```python
from build123d import *
from build123d.topology import SkipClean

# Parameters (mm, degrees)
ESQUISSE2_R             = 11
BOSS_EXTRU_1_DEPTH      = 20
ENL_V_START             = -10
ESQUISSE3_R             = 12
ESQUISSE3_R_2           = 11
ENL_V_MAT_EXTRU_1_DEPTH = 10
ESQUISSE4_W             = 3
ESQUISSE4_H             = 10
BOSS_EXTRU_2_DEPTH      = 4
ESQUISSE5_R             = 1.1
BOSS_EXTRU_3_DEPTH      = 1
ESQUISSE9_R             = 1.1
BOSS_EXTRU_5_DEPTH      = 2
BOSS_EXTRU_6_START      = -6
BOSS_EXTRU_6_DEPTH      = 8
CONG_1_R                = 1
CONG_2_R                = 1
BOSS_EXTRU_7_DEPTH      = 10
BOSS_EXTRU_8_DEPTH      = 10
BOSS_EXTRU_8_DEPTH_BACK = 5
CONG_3_R                = 10
CONG_4_R                = 3
ENL_V_MAT_EXTRU_2_REACH = 52.872
ESQUISSE11_R            = 3


with BuildPart() as part:
    # Esquisse2 → Boss.-Extru.1 (new body)
    with BuildSketch(Plane.XY):
        with BuildLine():
            Line((5.727272727, 12.774910845), (24.045454545, 4.562468159))
            ThreePointArc((24.045454545, 4.562468159), (27, 0), (24.045454545, -4.562468159))
            Line((24.045454545, -4.562468159), (5.727272727, -12.774910845))
            ThreePointArc((5.727272727, -12.774910845), (-14, 0), (5.727272727, 12.774910845))
        make_face()
        Circle(ESQUISSE2_R, mode=Mode.SUBTRACT)
    extrude(amount=BOSS_EXTRU_1_DEPTH)

    # Esquisse3 → Enlèv. mat.-Extru.1 (cut)
    with BuildSketch(Plane.XY.offset(20).offset(ENL_V_START)):
        Circle(ESQUISSE3_R)
        Circle(ESQUISSE3_R_2, mode=Mode.SUBTRACT)
    extrude(amount=ENL_V_MAT_EXTRU_1_DEPTH, mode=Mode.SUBTRACT)

    # Esquisse4 → Boss.-Extru.2 (add)
    with BuildSketch(Plane(origin=(5.727272727, -12.774910845, 0), x_dir=(0.9124936318129423, 0.4090909090909094, 0), z_dir=(0.40909090909090934, -0.9124936318129422, 0))):
        with Locations((17.5748599, 10)):
            Rectangle(ESQUISSE4_W, ESQUISSE4_H)
    extrude(amount=BOSS_EXTRU_2_DEPTH)

    # Esquisse5 → Boss.-Extru.3 (add)
    with BuildSketch(Plane.XY.offset(15)):
        with Locations(Location((22.582402284, -7.410182695, 0), (0, 0, 180))):
            Circle(ESQUISSE5_R)
    boss_extru_3 = extrude(amount=BOSS_EXTRU_3_DEPTH)

    # Symétrie1: Boss.-Extru.3 across plane
    add(boss_extru_3.mirror(Plane.XY.offset(10)))

    # Esquisse9 → Boss.-Extru.5 (add)
    # profile 1 of 2: a face of its own
    with BuildSketch(Plane.XY.offset(16)):
        with BuildLine():
            Line((21.323895477, -10.714144048), (23.605129557, -9.691416775))
            ThreePointArc((23.605129557, -9.691416775), (24.737785683, -6.717851558), (21.764220466, -5.585195432))
            Line((21.764220466, -5.585195432), (19.482986386, -6.607922705))
            Line((19.482986386, -6.607922705), (21.323895477, -10.714144048))
        make_face()
        with Locations(Location((22.582402284, -7.410182695, 0), (0, 0, 180))):
            Circle(ESQUISSE9_R, mode=Mode.SUBTRACT)
    # profile 2 of 2: a face of its own
    with BuildSketch(Plane.XY.offset(16)):
        with Locations(Location((22.582402284, -7.410182695, 0), (0, 0, 180))):
            Circle(ESQUISSE9_R)
    boss_extru_5 = extrude(amount=BOSS_EXTRU_5_DEPTH)

    # Esquisse9<4> → Boss.-Extru.6 (add)
    with BuildSketch(Plane.XY.offset(16).offset(BOSS_EXTRU_6_START)):
        with BuildLine():
            Line((-2.260153649, -21.287390546), (21.323895477, -10.714144048))
            Line((21.323895477, -10.714144048), (19.482986386, -6.607922705))
            Line((19.482986386, -6.607922705), (1.283727254, -14.767049742))
            ThreePointArc((1.283727254, -14.767049742), (0.201847525, -15.178661138), (-0.920349818, -15.462493505))
            Line((-0.920349818, -15.462493505), (-5.484659611, -16.339454049))
            ThreePointArc((-5.484659611, -16.339454049), (-7.55515779, -21.213423405), (-2.260153649, -21.287390546))
        make_face()
    boss_extru_6 = extrude(amount=BOSS_EXTRU_6_DEPTH)

    # Symétrie2: Boss.-Extru.5, Boss.-Extru.6 across plane
    add(boss_extru_5.mirror(Plane.XY.offset(10)))
    add(boss_extru_6.mirror(Plane.XY.offset(10)))

    # Congé1
    cong_1_edges = [part.edges().sort_by_distance(p)[0] for p in [
        (24.76932455, -8.621533595, 10),
    ]]
    fillet(cong_1_edges, radius=CONG_1_R)

    # Congé2
    cong_2_edges = [part.edges().sort_by_distance(p)[0] for p in [
        (22.031843655, -9.848806323, 10),
    ]]
    fillet(cong_2_edges, radius=CONG_2_R)

    # Esquisse10 → Boss.-Extru.7 (add)
    with SkipClean():  # the faces are left unmerged after this step: merging them gives an invalid solid
        with BuildSketch(Plane.XY.offset(20)):
            with BuildLine():
                Line((-13.651031791, -3.10633724), (-11.590973598, -3.10633724))
                ThreePointArc((-11.590973598, -3.10633724), (-12, 0), (-11.590973598, 3.10633724))
                Line((-11.590973598, 3.10633724), (-13.651031791, 3.10633724))
                ThreePointArc((-13.651031791, 3.10633724), (-14, 0), (-13.651031791, -3.10633724))
            make_face()
        extrude(amount=BOSS_EXTRU_7_DEPTH)

    # Esquisse10<3> → Boss.-Extru.8 (add, two sides: drawn at the far end of the back side and taken through both)
    with SkipClean():  # the faces are left unmerged after this step: merging them gives an invalid solid
        with BuildSketch(Plane.XY.offset(20).offset(-BOSS_EXTRU_8_DEPTH_BACK)):
            with BuildLine():
                Line((-32, -3.10633724), (-13.651031791, -3.10633724))
                ThreePointArc((-13.651031791, -3.10633724), (-13.912484413, -1.562938727), (-14, 0))
                ThreePointArc((-14, 0), (-13.912484413, 1.562938727), (-13.651031791, 3.10633724))
                Line((-13.651031791, 3.10633724), (-32, 3.10633724))
                Line((-32, 3.10633724), (-32, -3.10633724))
            make_face()
        extrude(amount=BOSS_EXTRU_8_DEPTH + BOSS_EXTRU_8_DEPTH_BACK)

    # Congé3
    cong_3_edges = [part.edges().sort_by_distance(p)[0] for p in [
        (-32, 0, 15),
    ]]
    fillet(cong_3_edges, radius=CONG_3_R)

    # Congé4
    cong_4_edges = [part.edges().sort_by_distance(p)[0] for p in [
        (-32, 0, 30),
    ]]
    fillet(cong_4_edges, radius=CONG_4_R)

    # Esquisse11 → Enlèv. mat.-Extru.2 (cut, up to next)
    with BuildSketch(Plane(origin=(0, 3.10633724, 0), x_dir=(1, 0, 0), z_dir=(0, 1, 0)), mode=Mode.PRIVATE) as enl_v_mat_extru_2_sk1:
        with Locations(Location((-28, -26, 0), (0, 0, 180))):
            Circle(ESQUISSE11_R)
    enl_v_mat_extru_2_tool1 = extrude(enl_v_mat_extru_2_sk1.sketch, amount=-ENL_V_MAT_EXTRU_2_REACH, mode=Mode.PRIVATE) & part.part
    add(enl_v_mat_extru_2_tool1.solids().sort_by_distance((-28, 3.106337, 26))[0], mode=Mode.SUBTRACT)


solid = part.part
```
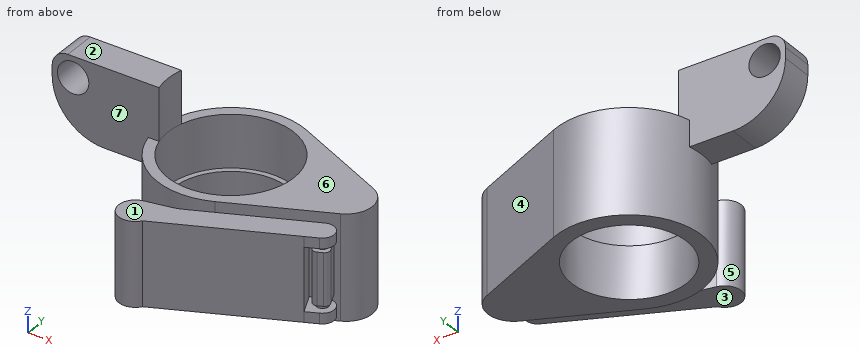
Model file for the job. Use its own axes, mm. Face numbers are marked on the shaded views. A direction names the side the tool comes from. Round coordinates to 2 decimals unless told otherwise and drop trailing zeros. Order: outer loops, then holes, each group sorted by start corner. A loop starts at its lowest first (then second) coordinate and runs counter-clockwise, first axis right, second up. Notation, with made-up numbers: (14, -4) -> (19, -4) arc R31 ccw to (19, 27) -> close; hole circle Ø4 at (10, -14.75). An arc over 180 degrees is marked (long way). Use one line per item in the form item = value.
Item 1: Pull direction Y, two halves, no side cores. Call the marked faces 4, 5, 6 and 7: released by +Y, released by -Y, zero draft, split by the parting line, or undercut.
Returned:
face_4 = released by +Y
face_5 = undercut
face_6 = zero draft
face_7 = released by -Y
Item 2: Cut at D-D, the plane x = -28. Write the cut outline in (y, z), and give its area (3 significant figures).
Returned:
outline = (-3.11, 17) -> (3.11, 17) -> (3.11, 23) -> (-3.11, 23) -> close; (-3.11, 29) -> (3.11, 29) -> (3.11, 30) -> (-3.11, 30) -> close
area = 43.5 mm^2
Item 3: Cut at A-A, the plane y = 0. Write the cut outline in (x, z).
Returned:
outline = (-32, 25) arc R10 ccw to (-22, 15) -> (-14, 15) -> (-14, 0) -> (-11, 0) -> (-11, 10) -> (-12, 10) -> (-12, 30) -> (-29, 30) arc R3 ccw to (-32, 27) -> close; (11, 0) -> (27, 0) -> (27, 20) -> (12, 20) -> (12, 10) -> (11, 10) -> close; hole circle Ø6 at (-28, 26)
Item 4: Drill centre lines: line 1 (Y direction, x = 0, z = 5.75); line 2 (Y direction, x = -6.5, z = 12.5); line 3 (Z direction, x = 12.5, y = 8). Where is each one in solid material? Low to high.
Returned:
line_1 = -20.27 to -15.24, -14 to -11, 11 to 14
line_2 = -22.22 to -16.72, -12.4 to -10.09, 10.09 to 12.4
line_3 = 0 to 20
Item 5: Flat gauge pins, fed straight in: pin 1 Ø1.2 at (x, y) = (22, -7) entering from -Z; pin 2 Ø5 at (y, z) = (0.5, 24) entering from +X; pin 3 Ø6 at (x, y) = (22.5, -7.5) entering from +Z. Where does each tip first touch, or does it go through?
Returned:
pin_1 = 2
pin_2 = -11.62
pin_3 = 20
Item 6: Cut at B-B, the plane z = 26. Write the cut outline in (x, y).
Returned:
outline = (-32, -3.11) -> (-31, -3.11) -> (-31, 3.11) -> (-32, 3.11) -> close; (-25, -3.11) -> (-11.59, -3.11) arc R12 cw to (-11.59, 3.11) -> (-25, 3.11) -> close
Item 7: Tool access for the marked faces 1, 2 and 3: list every direction of +Z, -Z, +X, -X, +Y, -Y with a clear straight run to the whole face (end or side of a thin tool).
Returned:
face_1 = +Z, +X, -Y
face_2 = +Z, +X, -X, +Y, -Y
face_3 = -Z, +X, -Y
Item 8: Cut at C-C, the plane z = 12.75. Write the cut outline in (x, y).
Returned:
outline = (-5.48, -16.34) arc R3.19 ccw (long way) to (-2.26, -21.29) -> (21.32, -10.71) -> (19.48, -6.61) -> (20.4, -6.2) -> (21.62, -8.94) arc R1 ccw to (22.94, -9.44) -> (23.86, -9.03) arc R1 ccw to (24.36, -7.71) -> (23.13, -4.97) -> (24.05, -4.56) arc R5 ccw to (24.05, 4.56) -> (5.73, 12.77) arc R14 ccw (long way) to (5.73, -12.77) -> (1.28, -14.77) arc R10 cw to (-0.92, -15.46) -> close; hole circle Ø24 at (0, 0)
